from build123d import *

# Parameters (mm, degrees)
PAD_DEPTH = 8
FILLET_R  = 3


with BuildPart() as part:
    # Sketch → Pad (new body)
    with BuildSketch(Plane.XY):
        with BuildLine():
            ThreePointArc((-25.332917, -7), (-11.2, 0), (-25.332917, 7))
            ThreePointArc((-27.75697, 10.181818), (-28.135852, 7.378883), (-25.332917, 7))
            ThreePointArc((-7.841053, 4), (-16.205521, 12.224644), (-27.75697, 10.181818))
            Line((0, 4), (-7.841053, 4))
            Line((0, 4), (7.841053, 4))
            ThreePointArc((27.75697, 10.181818), (16.205521, 12.224644), (7.841053, 4))
            ThreePointArc((25.332917, 7), (28.135852, 7.378883), (27.75697, 10.181818))
            ThreePointArc((25.332917, 7), (11.2, 0), (25.332917, -7))
            ThreePointArc((27.75697, -10.181818), (28.135852, -7.378883), (25.332917, -7))
            ThreePointArc((7.841053, -4), (16.205521, -12.224644), (27.75697, -10.181818))
            Line((0, -4), (7.841053, -4))
            Line((0, -4), (-7.841053, -4))
            ThreePointArc((-27.75697, -10.181818), (-16.205521, -12.224644), (-7.841053, -4))
            ThreePointArc((-25.332917, -7), (-28.135852, -7.378883), (-27.75697, -10.181818))
        make_face()
    extrude(amount=PAD_DEPTH)

    # Fillet
    fillet_edges = [part.edges().sort_by_distance(p)[0] for p in [
        (-7.841053, -4, 4),
        (7.841053, -4, 4),
        (-7.841053, 4, 4),
        (7.841053, 4, 4),
    ]]
    fillet(fillet_edges, radius=FILLET_R)


solid = part.part
Work out the finished part from the listing and answer in its coordinate system (mm). A direction names the side the tool comes from. Coordinates: 2 decimals unless noted, no trailing zeros. Write each loop counter-clockwise with the first axis right and the second up, starting at its lowest first coordinate (ties: lowest second). Pieces come first, ordered by that corner, then holes.
1. Consider line 1 along Y through (x, z) = (20, 2.75); line 2 along X through (y, z) = (6.75, 6); line 3 along Y through (x, z) = (-3, 3.5). Determine where each line is inside the solid, lowest interval first.
Results list:
line 1: y = -12.8 to -8.8, 8.8 to 12.8
line 2: x = -27.33 to -25.76, -14.35 to -9.12, 9.12 to 14.35, 25.76 to 27.33
line 3: y = -4 to 4
2. The part is cut by section D-D, the plane y = 0. Write down the section's boundary in (x, z).
Results list:
outline: (-11.2, 0) - (11.2, 0) - (11.2, 8) - (-11.2, 8) - close
3. The part is cut by section C-C, the plane y = 9.5. Write down the section's boundary in (x, z), and give its area (3 significant figures).
Results list:
outline: (-28.33, 0) - (-11.42, 0) - (-11.42, 8) - (-28.33, 8) - close; (11.42, 0) - (28.33, 0) - (28.33, 8) - (11.42, 8) - close
area: 270 mm2
4. For faces 1 (the flat face through (0, 4, 4)), 2 (the cylindrical face through (-7.4, -4.44, 4.06)), 3 (the cylindrical face through (-28.16, 7.41, 3.94)), determine the directions among +Z, -Z, +X, -X, +Y, -Y from which every point of the face is accessible in a straight line to the end or side of a thin tool.
Results list:
face 1: +Z, -Z, +Y
face 2: +Z, -Z, -Y
face 3: +Z, -Z
5. For a pull along Y with two mould halves and no side action, classify faces 4 (the cylindrical face through (11.204, 0.274, 3.944)), 5 (the cylindrical face through (28.16, -7.41, 3.94)), 6 (the flat face through (0, -4, 4)), 7 (the flat face through (0, 1, 0)) as +Y half, -Y half, draft (parallel to the pull), parting line (faces both ways), or undercut.
Results list:
face 4: undercut
face 5: undercut
face 6: -Y half
face 7: draft
6. The part is cut by section A-A, the plane x = -20. Write down the section's boundary in (y, z), and give its area (3 significant figures).
Results list:
outline: (-12.8, 0) - (-8.8, 0) - (-8.8, 8) - (-12.8, 8) - close; (8.8, 0) - (12.8, 0) - (12.8, 8) - (8.8, 8) - close
area: 64.0 mm2
7. The part is cut by section B-B, the plane z = 5.5. Write down the section's boundary in (x, y), and give its area (3 significant figures).
Results list:
outline: (-27.76, -10.18) arc R12.8 ccw to (-8.52, -5.67) arc R3 cw to (-5.84, -4) - (5.84, -4) arc R3 cw to (8.52, -5.67) arc R12.8 ccw to (27.76, -10.18) arc R2 ccw to (25.33, -7) arc R8.8 cw (long way) to (25.33, 7) arc R2 ccw to (27.76, 10.18) arc R12.8 ccw to (8.52, 5.67) arc R3 cw to (5.84, 4) - (-5.84, 4) arc R3 cw to (-8.52, 5.67) arc R12.8 ccw to (-27.76, 10.18) arc R2 ccw to (-25.33, 7) arc R8.8 cw (long way) to (-25.33, -7) arc R2 ccw to start
area: 530 mm2
8. Flat-ended cylindrical pins translate along their axes: pin 1 (2 mm diameter, centred on y = 5.5, z = 4, fed in from -X); pin 2 (2.5 mm diameter, centred on x = 2, z = 3, fed in from +Y); pin 3 (3 mm diameter, centred on x = 15.5, z = 3, fed in from +Y). Find the tip coordinate at first contact, or state that the pin passes through.
Results list:
pin 1: stops at x = -14.07
pin 2: stops at y = 4
pin 3: stops at y = 12.44
